The listing builds one solid part. Answer for the finished solid, in the listing's coordinates (mm). A direction names the side the tool comes from. Coordinates: 2 decimals unless noted, no trailing zeros. Loops run counter-clockwise (first coordinate to the right, second up) from the corner with the lowest first, then second, coordinate; pieces in that order, holes last. Notation, with made-up numbers: M 2,50.5 L 12,50.5 A4 ccw 12,56.5 Z; hole C 32.5,-10.5 d9. An arc over 180 degrees is marked long. Answer as a JSON object with one key per item and string values. Group by question number.
1. Straight lines are drawn through the part: L1, parallel to X at y = 6.25, z = 5.3; L2, parallel to Y at x = -6.4, z = 3; L3, parallel to Z at x = 7.8, y = 5. For each, find the intervals that lie inside material, in ascending order.
2. Determine the mould class of faces 6 (the face through (-5, 4, 4)), 7 (the face through (-4.43, 0.6, 3.04)), 8 (the face through (-6.972, 3.891, 2.423)) for opening direction Y: released by +Y, released by -Y, zero draft, split by the parting line, or undercut.
3. A cutting plane is placed at A-A on z = 3. Give the vertices of the cut face in (x, y).
4. Given pin 1 (1 mm diameter, centred on x = 6.5, y = -3, fed in from -Z); pin 2 (2 mm diameter, centred on y = 5, z = 3, fed in from +X); pin 3 (1.8 mm diameter, centred on y = 6, z = 4, fed in from +X); pin 4 (3 mm diameter, centred on y = 4.5, z = 3, fed in from -X), each flat-ended and moving along its own axis, determine where each tip first touches the part or whether it passes through.
5. A cutting plane is placed at C-C on y = 5. Give the vertices of the cut face in (x, z), and give its area (3 significant figures).
6. A cutting plane is placed at D-D on x = -6.25. Give the vertices of the cut face in (y, z), and give its area (3 significant figures).
7. For faces 1 (the face through (6.972, 3.891, 2.423)), 2 (the face through (-13, 0, 3)), 3 (the face through (4.43, 0.6, 3.04)), 4 (the face through (8.75, -2.95, 2.96)), 5 (the face through (9, 4, 4)), determine the directions among +Z, -Z, +X, -X, +Y, -Y from which every point of the face is accessible in a straight line to the end or side of a thin tool.
8. A cutting plane is placed at B-B on y = -3. Give the vertices of the cut face in (x, z).
from build123d import *

# Parameters (mm, degrees)
SKETCH_1_R               = 1.25
EXTRUDE_1_DEPTH          = 6
CHAMFER_1_SIZE           = 2
SKETCH_2_R               = 1.25
CUT_EXTRUDE_1_DEPTH      = 16
CUT_EXTRUDE_1_DEPTH_BACK = 16
FILLET_1_R               = 2


with BuildPart() as part:
    # 草图1 → 凸台-拉伸1 (new body)
    with BuildSketch(Plane.XY):
        Polygon((-15, -6), (15, -6), (15, 0), (9, 0), (9, 8), (5, 8), (5, 0), (-5, 0), (-5, 8), (-9, 8), (-9, 0), (-15, 0), align=None)
        with Locations((-10, -3)):
            Circle(SKETCH_1_R, mode=Mode.SUBTRACT)
        with Locations((10, -3)):
            Circle(SKETCH_1_R, mode=Mode.SUBTRACT)
    extrude(amount=EXTRUDE_1_DEPTH)

    # 倒角1
    chamfer_1_edges = [part.edges().sort_by_distance(p)[0] for p in [
        (-7, 8, 0),
        (7, 8, 0),
    ]]
    chamfer(chamfer_1_edges, length=CHAMFER_1_SIZE)

    # 草图2 → 切除-拉伸1 (cut, two sides)
    with BuildSketch(Plane(origin=(0, 0, 0), x_dir=(0, 0, -1), z_dir=(1, 0, 0))) as cut_extrude_1_sk:
        with Locations((-3, 5)):
            Circle(SKETCH_2_R)
    extrude(amount=CUT_EXTRUDE_1_DEPTH, mode=Mode.SUBTRACT)
    extrude(cut_extrude_1_sk.sketch, amount=-CUT_EXTRUDE_1_DEPTH_BACK, mode=Mode.SUBTRACT)

    # 圆角1
    fillet_1_edges = [part.edges().sort_by_distance(p)[0] for p in [
        (-9, 0, 3),
        (-5, 0, 3),
        (5, 0, 3),
        (9, 0, 3),
    ]]
    fillet(fillet_1_edges, radius=FILLET_1_R)


solid = part.part
From the geometry:
{
 "1": {"L1": "x = -9 to -5, 5 to 9", "L2": "y = -6 to 3.75, 6.25 to 8", "L3": "z = 0 to 1.75, 4.25 to 6"},
 "2": {"face 6": "zero draft", "face 7": "released by +Y", "face 8": "undercut"},
 "3": {"outline": "M -15,-6 L 15,-6 L 15,0 L 11,0 A2 cw 9,2 L 9,3.75 L 5,3.75 L 5,2 A2 cw 3,0 L -3,0 A2 cw -5,2 L -5,3.75 L -9,3.75 L -9,2 A2 cw -11,0 L -15,0 Z; M -9,6.25 L -5,6.25 L -5,8 L -9,8 Z; M 5,6.25 L 9,6.25 L 9,8 L 5,8 Z; hole C -10,-3 d2.5; hole C 10,-3 d2.5"},
 "4": {"pin 1": "stops at z = 0", "pin 2": "passes through", "pin 3": "stops at x = 9", "pin 4": "stops at x = -9"},
 "5": {"outline": "M -9,0 L -5,0 L -5,1.75 L -9,1.75 Z; M -9,4.25 L -5,4.25 L -5,6 L -9,6 Z; M 5,0 L 9,0 L 9,1.75 L 5,1.75 Z; M 5,4.25 L 9,4.25 L 9,6 L 5,6 Z", "area": "28.0 mm²"},
 "6": {"outline": "M -6,0 L 6,0 L 8,2 L 8,6 L -6,6 Z; hole C 5,3 d2.5", "area": "77.1 mm²"},
 "7": {"face 1": "+X, -X", "face 2": "+Z, -Z, -X, +Y", "face 3": "+Z, -Z, +Y", "face 4": "+Z, -Z", "face 5": "+Z, -Z, +X, +Y"},
 "8": {"outline": "M -15,0 L -11.25,0 L -11.25,6 L -15,6 Z; M -8.75,0 L 8.75,0 L 8.75,6 L -8.75,6 Z; M 11.25,0 L 15,0 L 15,6 L 11.25,6 Z"}
}
